```python
from build123d import *

# Parameters (mm, degrees)
CROQUIS1_W               = 38
CROQUIS1_H               = 81
CROQUIS1_W_2             = 27
CROQUIS1_H_2             = 72
CROQUIS1_H_3             = 38
CROQUIS1_R               = 3.5
SALIENTE_EXTRUIR1_DEPTH  = 5
CROQUIS2_W               = 38
CROQUIS2_H               = 81
CROQUIS2_W_2             = 27
CROQUIS2_H_2             = 72
SALIENTE_EXTRUIR2_DEPTH  = 5
SALIENTE_EXTRUIR9_START  = -1
SALIENTE_EXTRUIR9_DEPTH  = 1
SALIENTE_EXTRUIR10_DEPTH = 11
SALIENTE_EXTRUIR11_DEPTH = 10
REDONDEO1_R              = 1
REDONDEO2_R              = 1
REDONDEO3_R              = 1
CROQUIS6_W               = 6
CROQUIS6_H               = 9
CORTAR_EXTRUIR1_DEPTH    = 8
CROQUIS7_W               = 6
CROQUIS7_H               = 9
CROQUIS7_R               = 2.5
SALIENTE_EXTRUIR12_DEPTH = 3
SALIENTE_EXTRUIR13_DEPTH = 11
REDONDEO4_R              = 5
CROQUIS9_R               = 0.6
CORTAR_EXTRUIR2_DEPTH    = 80
SALIENTE_EXTRUIR14_START = -2.5
CROQUIS10_R              = 0.6
SALIENTE_EXTRUIR14_DEPTH = 2.5
CROQUIS11_R              = 4
CROQUIS11_R_2            = 3.5
CROQUIS11_R_3            = 2.5
CROQUIS11_R_4            = 2
CORTAR_EXTRUIR3_DEPTH    = 1
SALIENTE_EXTRUIR15_DEPTH = 3
CROQUIS14_R              = 1.5
CORTAR_EXTRUIR4_DEPTH    = 14
CROQUIS16_W              = 3.5
CROQUIS16_H              = 3
SALIENTE_EXTRUIR16_DEPTH = 4
CROQUIS25_R              = 3
CROQUIS25_R_2            = 1.5
SALIENTE_EXTRUIR21_DEPTH = 18
CROQUIS26_R              = 1.5
CORTAR_EXTRUIR7_DEPTH    = 18
CROQUIS28_R              = 1
CORTAR_EXTRUIR8_DEPTH    = 4
CROQUIS29_W              = 16
CROQUIS29_H              = 4
CORTAR_EXTRUIR9_DEPTH    = 5


with BuildPart() as part:
    # Croquis1 → Saliente-Extruir1 (new body)
    # profile 1 of 5: a face of its own
    with BuildSketch(Plane.XY):
        Rectangle(CROQUIS1_W, CROQUIS1_H)
        Rectangle(CROQUIS1_W_2, CROQUIS1_H_2, mode=Mode.SUBTRACT)
    # profile 2 of 5: a face of its own
    with BuildSketch(Plane.XY):
        with Locations((0, -59.5)):
            Rectangle(CROQUIS1_W, CROQUIS1_H_3)
        with Locations((-9.5, -69)):
            Circle(CROQUIS1_R, mode=Mode.SUBTRACT)
        with Locations((9.5, -59.5)):
            Circle(CROQUIS1_R, mode=Mode.SUBTRACT)
        with Locations((-9.5, -50)):
            Circle(CROQUIS1_R, mode=Mode.SUBTRACT)
    # profile 3 of 5: a face of its own
    with BuildSketch(Plane.XY):
        with BuildLine():
            ThreePointArc((19, -78.5), (26.870057685, -59.5), (19, -40.5))
            Line((19, -40.5), (19, -78.5))
        make_face()
    # profile 4 of 5: a face of its own
    with BuildSketch(Plane.XY):
        with BuildLine():
            Line((19, -78.5), (-19, -78.5))
            ThreePointArc((-19, -78.5), (0, -86.370057685), (19, -78.5))
        make_face()
    # profile 5 of 5: a face of its own
    with BuildSketch(Plane.XY):
        with BuildLine():
            Line((-19, -78.5), (-19, -40.5))
            ThreePointArc((-19, -40.5), (-26.870057685, -59.5), (-19, -78.5))
        make_face()
    extrude(amount=SALIENTE_EXTRUIR1_DEPTH)

    # Croquis2 → Saliente-Extruir2 (add)
    with BuildSketch(Plane(origin=(0, 0, 0), x_dir=(-1, 0, 0), z_dir=(0, 0, -1))):
        Rectangle(CROQUIS2_W, CROQUIS2_H)
        Rectangle(CROQUIS2_W_2, CROQUIS2_H_2, mode=Mode.SUBTRACT)
    extrude(amount=SALIENTE_EXTRUIR2_DEPTH)

    # Croquis3 → Saliente-Extruir9 (add)
    with BuildSketch(Plane.XY.offset(5).offset(SALIENTE_EXTRUIR9_START)):
        with BuildLine():
            Line((26.870057685, -59.5), (26.870057685, 40.5))
            Line((26.870057685, 40.5), (19, 48.370057685))
            Line((19, 48.370057685), (-19, 48.370057685))
            Line((-19, 48.370057685), (-26.870057685, 40.5))
            Line((-26.870057685, 40.5), (-26.870057685, -59.5))
            ThreePointArc((-26.870057685, -59.5), (0, -86.370057685), (26.870057685, -59.5))
        make_face()
        with BuildLine():
            Line((19, -59.5), (19, 40.5))
            Line((19, 40.5), (-19, 40.5))
            Line((-19, 40.5), (-19, -59.5))
            ThreePointArc((-19, -59.5), (0, -78.5), (19, -59.5))
        make_face(mode=Mode.SUBTRACT)
    extrude(amount=SALIENTE_EXTRUIR9_DEPTH)

    # Croquis4 → Saliente-Extruir10 (add)
    with BuildSketch(Plane(origin=(0, 0, 4), x_dir=(-1, 0, 0), z_dir=(0, 0, -1))):
        with BuildLine():
            Line((19, 40.5), (19, -40.5))
            ThreePointArc((19, -40.5), (24.824696333, -49.217274097), (26.870057685, -59.5))
            Line((26.870057685, -59.5), (26.870057685, 40.5))
            Line((26.870057685, 40.5), (19, 48.370057685))
            Line((19, 48.370057685), (-19, 48.370057685))
            Line((-19, 48.370057685), (-26.870057685, 40.5))
            Line((-26.870057685, 40.5), (-26.870057685, -59.5))
            ThreePointArc((-26.870057685, -59.5), (-24.824696333, -49.217274097), (-19, -40.5))
            Line((-19, -40.5), (-19, 40.5))
            Line((-19, 40.5), (19, 40.5))
        make_face()
    extrude(amount=-SALIENTE_EXTRUIR10_DEPTH)

    # Croquis5 → Saliente-Extruir11 (add)
    with BuildSketch(Plane.XY.offset(5)):
        with BuildLine():
            Line((-19, -59.5), (-19, -69))
            ThreePointArc((-19, -69), (-16.217514421, -75.717514421), (-9.5, -78.5))
            Line((-9.5, -78.5), (9.5, -78.5))
            ThreePointArc((9.5, -78.5), (16.217514421, -75.717514421), (19, -69))
            Line((19, -69), (19, -59.5))
            Line((19, -59.5), (19, -40.5))
            ThreePointArc((19, -40.5), (0, -86.370057685), (-19, -40.5))
            Line((-19, -40.5), (-19, -59.5))
        make_face()
    extrude(amount=SALIENTE_EXTRUIR11_DEPTH)

    # Redondeo1
    redondeo1_edges = [part.edges().sort_by_distance(p)[0] for p in [
        (19, -40.5, -2.5),
        (-19, -40.5, -2.5),
        (19, 40.5, -0.5),
        (-19, 40.5, -0.5),
    ]]
    fillet(redondeo1_edges, radius=REDONDEO1_R)

    # Redondeo2
    redondeo2_edges = [part.edges().sort_by_distance(p)[0] for p in [
        (-19, -0.5, 4),
        (0, 40.5, 4),
        (-18.707106781, 40.207106781, 4),
        (18.707106781, 40.207106781, 4),
        (19, -0.5, 4),
    ]]
    fillet(redondeo2_edges, radius=REDONDEO2_R)

    # Redondeo3
    redondeo3_edges = [part.edges().sort_by_distance(p)[0] for p in [
        (19, 48.370057685, 9.5),
        (26.870057685, 40.5, 9.5),
        (-26.870057685, 40.5, 9.5),
        (-19, 48.370057685, 9.5),
    ]]
    fillet(redondeo3_edges, radius=REDONDEO3_R)

    # Croquis6 → Cortar-Extruir1 (cut)
    with BuildSketch(Plane.ZY.offset(26.870057685)):
        with Locations((11.5, -55)):
            Rectangle(CROQUIS6_W, CROQUIS6_H)
    extrude(amount=-CORTAR_EXTRUIR1_DEPTH, mode=Mode.SUBTRACT)

    # Croquis7 → Saliente-Extruir12 (add)
    with BuildSketch(Plane.ZY.offset(26.870057685)):
        with Locations((11.5, -55)):
            Rectangle(CROQUIS7_W, CROQUIS7_H)
        with Locations((11.5, -55)):
            Circle(CROQUIS7_R, mode=Mode.SUBTRACT)
    extrude(amount=-SALIENTE_EXTRUIR12_DEPTH)

    # Croquis8 → Saliente-Extruir13 (add)
    with BuildSketch(Plane.ZY.offset(26.870057685)):
        Polygon((15, 40.085786438), (4, 40.085786438), (4, 37.085786438), (9.5, 37.085786438), (15, 37.085786438), align=None)
        Polygon((9.5, 15.085786438), (4, 15.085786438), (4, 12.085786438), (9.5, 12.085786438), (15, 12.085786438), (15, 15.085786438), align=None)
        Polygon((9.5, -10.914213562), (4, -10.914213562), (4, -13.914213562), (9.5, -13.914213562), (15, -13.914213562), (15, -10.914213562), align=None)
        Polygon((9.5, -36.914213562), (4, -36.914213562), (4, -39.914213562), (15, -39.914213562), (15, -36.914213562), align=None)
    extrude(amount=SALIENTE_EXTRUIR13_DEPTH)

    # Redondeo4
    redondeo4_edges = [part.edges().sort_by_distance(p)[0] for p in [
        (-37.870057685, 38.585786438, 4),
        (-37.870057685, 38.585786438, 15),
        (-37.870057685, 13.585786438, 4),
        (-37.870057685, 13.585786438, 15),
        (-37.870057685, -12.414213562, 4),
        (-37.870057685, -12.414213562, 15),
        (-37.870057685, -38.414213562, 4),
        (-37.870057685, -38.414213562, 15),
    ]]
    fillet(redondeo4_edges, radius=REDONDEO4_R)

    # Croquis9 → Cortar-Extruir2 (cut)
    with BuildSketch(Plane(origin=(0, 40.085786438, 0), x_dir=(1, 0, 0), z_dir=(0, 1, 0))):
        with Locations(Location((-32.370057685, -9.5, 0), (0, 0, 270))):
            Circle(CROQUIS9_R)
    extrude(amount=-CORTAR_EXTRUIR2_DEPTH, mode=Mode.SUBTRACT)

    # Croquis10 → Saliente-Extruir14 (add)
    with BuildSketch(Plane.XZ.offset(39.914213562).offset(SALIENTE_EXTRUIR14_START)):
        with Locations(Location((-32.370057685, 9.5, 0), (0, 0, 90))):
            Circle(CROQUIS10_R)
    extrude(amount=SALIENTE_EXTRUIR14_DEPTH)

    # Croquis11 → Cortar-Extruir3 (cut)
    # profile 1 of 2: a face of its own
    with BuildSketch(Plane(origin=(0, -36.914213562, 0), x_dir=(1, 0, 0), z_dir=(0, 1, 0))):
        with Locations(Location((-32.370057685, -9.5, 0), (0, 0, 270))):
            Circle(CROQUIS11_R)
        with Locations(Location((-32.370057685, -9.5, 0), (0, 0, 270))):
            Circle(CROQUIS11_R_2, mode=Mode.SUBTRACT)
    # profile 2 of 2: a face of its own
    with BuildSketch(Plane(origin=(0, -36.914213562, 0), x_dir=(1, 0, 0), z_dir=(0, 1, 0))):
        with Locations(Location((-32.370057685, -9.5, 0), (0, 0, 270))):
            Circle(CROQUIS11_R_3)
        with Locations(Location((-32.370057685, -9.5, 0), (0, 0, 270))):
            Circle(CROQUIS11_R_4, mode=Mode.SUBTRACT)
    extrude(amount=-CORTAR_EXTRUIR3_DEPTH, mode=Mode.SUBTRACT)

    # Croquis13 → Saliente-Extruir15 (add)
    with BuildSketch(Plane.XY.offset(15)):
        Polygon((-19, -65.5), (-19, 40.5), (-22.5, 40.5), (-22.5, -69), (-19, -69), align=None)
        Polygon((22.5, 40.5), (19, 40.5), (19, -65.5), (19, -69), (22.5, -69), align=None)
        with BuildLine():
            Line((-19, 40.5), (19, 40.5))
            Line((19, 40.5), (22.5, 40.5))
            Line((22.5, 40.5), (22.5, 44.870057685))
            Line((22.5, 44.870057685), (19.292893219, 48.077164466))
            ThreePointArc((19.292893219, 48.077164466), (18.96846987, 48.293937218), (18.585786438, 48.370057685))
            Line((18.585786438, 48.370057685), (-18.585786438, 48.370057685))
            ThreePointArc((-18.585786438, 48.370057685), (-18.96846987, 48.293937218), (-19.292893219, 48.077164466))
            Line((-19.292893219, 48.077164466), (-22.5, 44.870057685))
            Line((-22.5, 44.870057685), (-22.5, 40.5))
            Line((-22.5, 40.5), (-19, 40.5))
        make_face()
    extrude(amount=SALIENTE_EXTRUIR15_DEPTH)

    # Croquis14 → Cortar-Extruir4 (cut)
    with BuildSketch(Plane(origin=(0, 0, 4), x_dir=(-1, 0, 0), z_dir=(0, 0, -1))):
        with Locations((10, 45.370057685)):
            Circle(CROQUIS14_R)
        with Locations(Location((-10, 45.370057685, 0), (0, 0, 180))):
            Circle(CROQUIS14_R)
    extrude(amount=-CORTAR_EXTRUIR4_DEPTH, mode=Mode.SUBTRACT)

    # Croquis16 → Saliente-Extruir16 (add)
    with BuildSketch(Plane(origin=(0, -69, 0), x_dir=(-1, 0, 0), z_dir=(0, -1, 0))):
        with Locations((20.75, -16.5)):
            Rectangle(CROQUIS16_W, CROQUIS16_H)
        with Locations((-20.75, -16.5)):
            Rectangle(CROQUIS16_W, CROQUIS16_H)
    extrude(amount=SALIENTE_EXTRUIR16_DEPTH)

    # Croquis25 → Saliente-Extruir21 (add)
    with BuildSketch(Plane.XY.offset(18)):
        with Locations((0, -70.629942315)):
            Circle(CROQUIS25_R)
        with Locations((0, -70.629942315)):
            Circle(CROQUIS25_R_2, mode=Mode.SUBTRACT)
    extrude(amount=-SALIENTE_EXTRUIR21_DEPTH)

    # Croquis26 → Cortar-Extruir7 (cut)
    with BuildSketch(Plane.XY.offset(18)):
        with Locations((0, -70.629942315)):
            Circle(CROQUIS26_R)
    extrude(amount=-CORTAR_EXTRUIR7_DEPTH, mode=Mode.SUBTRACT)

    # Croquis28 → Cortar-Extruir8 (cut)
    with BuildSketch(Plane.XY.offset(5)):
        with Locations((-16.5, 38)):
            Circle(CROQUIS28_R)
        with Locations((14.5, 38)):
            Circle(CROQUIS28_R)
        with Locations((14.5, -37)):
            Circle(CROQUIS28_R)
        with Locations((-16.5, -37)):
            Circle(CROQUIS28_R)
    extrude(amount=-CORTAR_EXTRUIR8_DEPTH, mode=Mode.SUBTRACT)

    # Croquis29 → Cortar-Extruir9 (cut)
    with BuildSketch(Plane.XY.offset(5)):
        with Locations((2, -42.5)):
            Rectangle(CROQUIS29_W, CROQUIS29_H)
    extrude(amount=-CORTAR_EXTRUIR9_DEPTH, mode=Mode.SUBTRACT)


solid = part.part
```
Geometry: final body of the model. Coordinates: model frame, mm. A direction names the side the tool comes from. Round coordinates to 2 decimals unless told otherwise and drop trailing zeros. Loops run counter-clockwise (first coordinate to the right, second up) from the corner with the lowest first, then second, coordinate; pieces in that order, holes last. Notation, with made-up numbers: (-18, 53) -> (-1, 53) arc R25 cw to (-1, 88) -> close; hole circle Ø4 at (-2.75, 53.5). An arc over 180 degrees is marked (long way). Use one line per item in the form item = value.
Item 1: Material intervals for probe 1 along X at (y, z) = (-37.45, 9.5); probe 2 along X at (y, z) = (-12.7, 9.5); probe 3 along Y at (x, z) = (-32, 8.5), sorted ascending.
Evaluation:
probe_1 = -37.87 to -36.37, -35.87 to -34.87, -34.37 to -30.37, -29.87 to -28.87, -28.37 to -19, 19 to 26.87
probe_2 = -37.87 to -32.97, -31.77 to -19, 19 to 26.87
probe_3 = -39.91 to -36.91, -13.91 to -10.91, 12.09 to 15.09, 37.09 to 40.09
Item 2: Contact query for flat-ended pins moving along their axis: pin 1 Ø10.5 at (x, z) = (-4, 10.5) entering from -Y; pin 2 Ø1 at (x, z) = (18, 7) entering from -Y; pin 3 Ø1.8 at (x, y) = (-10, 45.37) entering from -Z; pin 4 Ø12 at (x, z) = (-31.5, 7) entering from +Y. Output: stop coordinate, or through.
Evaluation:
pin_1 = -86.37
pin_2 = -79.89
pin_3 = through
pin_4 = 41.87
Item 3: Cut plane A-A on y = -18. Output: boundary loops of the cut face in (x, z), then the cut area to 3 significant figures.
Evaluation:
outline = (-26.87, 4) -> (-20, 4) arc R1 cw to (-19, 3) -> (-19, -5) -> (-13.5, -5) -> (-13.5, 5) -> (-19, 5) -> (-19, 18) -> (-22.5, 18) -> (-22.5, 15) -> (-26.87, 15) -> close; (13.5, -5) -> (19, -5) -> (19, 3) arc R1 cw to (20, 4) -> (26.87, 4) -> (26.87, 15) -> (22.5, 15) -> (22.5, 18) -> (19, 18) -> (19, 5) -> (13.5, 5) -> close
area = 305 mm2
Item 4: Cut plane B-B on x = 0. Output: boundary loops of the cut face in (y, z), then the cut area to 3 significant figures.
Evaluation:
outline = (-86.37, 0) -> (-72.13, 0) -> (-72.13, 18) -> (-73.63, 18) -> (-73.63, 5) -> (-78.5, 5) -> (-78.5, 15) -> (-86.37, 15) -> close; (-69.13, 0) -> (-44.5, 0) -> (-44.5, 5) -> (-67.63, 5) -> (-67.63, 18) -> (-69.13, 18) -> close; (-40.5, -5) -> (-36, -5) -> (-36, 5) -> (-40.5, 5) -> close; (36, -5) -> (40.5, -5) -> (40.5, 3) arc R1 cw to (41.5, 4) -> (48.37, 4) -> (48.37, 18) -> (40.5, 18) -> (40.5, 5) -> (36, 5) -> close
area = 512 mm2
Item 5: Access query for faces 4 (the flat face through (2, -44.5, 3)), 5 (the flat face through (-32, -39.914, 9)), 6 (the flat face through (-21, 7, 4)), 7 (the flat face through (-21, -55, 8.5)). Directions: +Z, -Z, +X, -X, +Y, -Y. A direction counts if a zero-diameter tool reaches every point of the face in a straight line with its end or side. Return the directions, or none.
Evaluation:
face_4 = +Z, -Z
face_5 = +Z, -Z, -X, -Y
face_6 = -Z, +Y
face_7 = none
Item 6: Draft query along Y for faces 1 (the flat face through (-31, 40.086, 10)), 2 (the cylindrical face through (-16.291, -75.643, 9.93)), 3 (the cylindrical face through (-36.37, -12.39, 13.57)). Return one class per face: released by +Y, released by -Y, zero draft, split by the parting line, or undercut.
Evaluation:
face_1 = released by +Y
face_2 = undercut
face_3 = zero draft
